The model under review builds one solid part; all positions refer to its coordinate system, in mm. A direction names the side the tool comes from. Give positions to 0.01 mm unless a question says otherwise; leave off trailing zeros. Write each loop counter-clockwise with the first axis right and the second up, starting at its lowest first coordinate (ties: lowest second). Pieces come first, ordered by that corner, then holes. Notation, with made-up numbers: M 81,76 L 99,76 A24 cw 99,93 Z; hole C 24,63 d10. An arc over 180 degrees is marked long. Write each question's results on one line, items separated by ' | '. Start each with the question number.
from build123d import *

# Parameters (mm, degrees)
SKETCH1_W          = 22.1
SKETCH1_H          = 19.9
EXTRUDE1_DEPTH     = 3.175
SKETCH2_R          = 1.03251
EXTRUDE2_DEPTH     = 12.7
SKETCH4_R          = 1.25
CUT_EXTRUDE1_DEPTH = 7.35


with BuildPart() as part:
    # Sketch1 → Extrude1 (new body, symmetric)
    with BuildSketch(Plane.XY):
        Rectangle(SKETCH1_W, SKETCH1_H)
    extrude(amount=EXTRUDE1_DEPTH, both=True)

    # Sketch2 → Extrude2 (cut)
    with BuildSketch(Plane.XZ.offset(9.95)):
        with Locations(Location((0, 0, 0), (0, 0, 270))):  # turned: the seam where the file's is
            Circle(SKETCH2_R)
    extrude(amount=-EXTRUDE2_DEPTH, mode=Mode.SUBTRACT)

    # Sketch4 → Cut-Extrude1 (cut, through all)
    with BuildSketch(Plane.XY.offset(3.175)):
        with Locations((8.49, -5.19)):
            Circle(SKETCH4_R)
        with Locations((-8.51, 7.41)):
            Circle(SKETCH4_R)
        with Locations((8.51, 7.41)):
            Circle(SKETCH4_R)
        with Locations((-8.49, -5.19)):
            Circle(SKETCH4_R)
    extrude(amount=-CUT_EXTRUDE1_DEPTH, mode=Mode.SUBTRACT)


solid = part.part
(1) Clearance check with flat-ended pins moving along their axes: P1, Ø2, axis at x = -8.49, y = -5.19, coming from the -Z side; P2, Ø0.6, axis at x = 0.5, z = 0, coming from the -Y side. State where each tip first meets the part, or that it passes through.
(2) Add section C-C (z = 0). State the section outline as (x, y) points.
(3) Draft analysis for pull direction Z (two halves, no side actions). For faces 3 (the cylindrical face through (-7.913, -6.299, 0.044)), 4 (the flat face through (0, 2.75, 0)), 5 (the flat face through (0, 0, 3.175)), state which applies: pulls with the +Z half, pulls with the -Z half, needs draft (parallel to the pull), parting line crosses it, or undercut.
(4) Wall thickness on L1, parallel to Y at x = -8.49, z = 0.25; L2, parallel to X at y = -4.75, z = 0; L3, parallel to X at y = -8.25, z = 0: over which ranges is each line inside the solid? List them lowest first.
(5) Machinability: for faces 1 (the flat face through (0, 9.95, 0)), 2 (the cylindrical face through (-0.63, -3.69, 0.82)), which of the approach directions +Z, -Z, +X, -X, +Y, -Y give a long, thin tool a straight path to every point of the face, cutting with its end or side? Answer none if there is none.
(6) Add section D-D (x = -8.49). State the section outline as (y, z) points (3 decimals).
(7) Add section A-A (y = -5.19). Give the number of separate pieces and of enclosed holes in the cut face, then the cut area to 3 significant figures.
Calculated:
1) P1: passes through | P2: stops at y = 2.75
2) outline: M -11.05,-9.95 L -1.03,-9.95 L -1.03,2.75 L 1.03,2.75 L 1.03,-9.95 L 11.05,-9.95 L 11.05,9.95 L -11.05,9.95 Z; hole C -8.51,7.41 d2.5; hole C -8.49,-5.19 d2.5; hole C 8.49,-5.19 d2.5; hole C 8.51,7.41 d2.5
3) face 3: needs draft | face 4: undercut | face 5: pulls with the +Z half
4) L1: y = -9.95 to -6.44, -3.94 to 6.16, 8.66 to 9.95 | L2: x = -11.05 to -9.66, -7.32 to -1.03, 1.03 to 7.32, 9.66 to 11.05 | L3: x = -11.05 to -1.03, 1.03 to 11.05
5) face 1: +Z, -Z, +X, -X, +Y | face 2: -Y
6) outline: M -9.95,-3.175 L -6.44,-3.175 L -6.44,3.175 L -9.95,3.175 Z; M -3.94,-3.175 L 6.16,-3.175 L 6.16,3.175 L -3.94,3.175 Z; M 8.66,-3.175 L 9.95,-3.175 L 9.95,3.175 L 8.66,3.175 Z
7) separate pieces: 3 | enclosed holes: 1 | area: 105 mm²
